CAD build for the part. Positions are in the model's coordinates, mm. A direction names the side the tool comes from. Give positions to 0.01 mm unless a question says otherwise; leave off trailing zeros. Loops run counter-clockwise (first coordinate to the right, second up) from the corner with the lowest first, then second, coordinate; pieces in that order, holes last. Notation, with made-up numbers: (13, 50.25) - (57, 50.25) arc R25 ccw to (57, 69.25) - close; hole circle Ø6 at (50.25, -31.75). An arc over 180 degrees is marked (long way). Return JSON: item names as keys, results as strings.
from build123d import *

# Parameters (mm, degrees)
SKETCH1_W           = 85
SKETCH1_H           = 76.5
SKETCH1_R           = 1.5
BOSS_EXTRUDE1_DEPTH = 10
SKETCH2_W           = 7
SKETCH2_H           = 7
BOSS_EXTRUDE2_DEPTH = 10


with BuildPart() as part:
    # Sketch1 → Boss-Extrude1 (new body)
    with BuildSketch(Plane(origin=(0, 0, 0), x_dir=(1, 0, 0), z_dir=(0, 1, 0))):
        Rectangle(SKETCH1_W, SKETCH1_H)
        with Locations(Location((-29.5, 25.25, 0), (0, 0, 270))):
            Circle(SKETCH1_R, mode=Mode.SUBTRACT)
        with Locations(Location((-29.5, -25.25, 0), (0, 0, 270))):
            Circle(SKETCH1_R, mode=Mode.SUBTRACT)
        with Locations(Location((29.5, -25.25, 0), (0, 0, 270))):
            Circle(SKETCH1_R, mode=Mode.SUBTRACT)
        with Locations(Location((29.5, 25.25, 0), (0, 0, 270))):
            Circle(SKETCH1_R, mode=Mode.SUBTRACT)
    extrude(amount=BOSS_EXTRUDE1_DEPTH)

    # Sketch2 → Boss-Extrude2 (add)
    with BuildSketch(Plane(origin=(0, 10, 0), x_dir=(1, 0, 0), z_dir=(0, 1, 0))):
        with Locations((-39, 34.75)):
            Rectangle(SKETCH2_W, SKETCH2_H)
        with Locations((39, 34.75)):
            Rectangle(SKETCH2_W, SKETCH2_H)
        with Locations((-39, -34.75)):
            Rectangle(SKETCH2_W, SKETCH2_H)
        with Locations((39, -34.75)):
            Rectangle(SKETCH2_W, SKETCH2_H)
    extrude(amount=BOSS_EXTRUDE2_DEPTH)


solid = part.part
1. Drop flat-ended pins along their axis: P1, Ø3, axis at y = 13, z = 18, coming from the -X side; P2, Ø3.5, axis at x = -29.5, z = 25.25, coming from the +Y side; P3, Ø10, axis at x = -8.5, z = 15, coming from the -Y side. Give the stop position or say it passes through.
Values follow:
{"P1": "passes through", "P2": "stops at y = 10", "P3": "stops at y = 0"}
2. Pull direction Z, two halves, no side cores. Call faces 1 (the face through (-1, 8, 38.25)), 2 (the face through (30.51, 4.93, -26.36)), 3 (the face through (-39, 15, -31.25)), 4 (the face through (-39, 20, -35)): +Z half, -Z half, draft (parallel to the pull), parting line (faces both ways), or undercut.
Values follow:
{"face 1": "+Z half", "face 2": "undercut", "face 3": "undercut", "face 4": "draft"}
3. Cut at C-C, the plane x = 29.5. Write the cut outline in (y, z), plus the area to 3 significant figures.
Values follow:
{"outline": "(0, -38.25) - (10, -38.25) - (10, -26.75) - (0, -26.75) - close; (0, -23.75) - (10, -23.75) - (10, 23.75) - (0, 23.75) - close; (0, 26.75) - (10, 26.75) - (10, 38.25) - (0, 38.25) - close", "area": "705 mm²"}
4. Drill centre lines: probe 1 along X at (y, z) = (6.75, -25.25); probe 2 along Y at (x, z) = (22, -23); probe 3 along X at (y, z) = (3.5, 24). Where is each one in solid material? Low to high.
Values follow:
{"probe 1": "x = -42.5 to -31, -28 to 28, 31 to 42.5", "probe 2": "y = 0 to 10", "probe 3": "x = -42.5 to -30.33, -28.67 to 28.67, 30.33 to 42.5"}
5. Cut at B-B, the plane z = -25.25. Write the cut outline in (x, y), plus the area to 3 significant figures.
Values follow:
{"outline": "(-42.5, 0) - (-31, 0) - (-31, 10) - (-42.5, 10) - close; (-28, 0) - (28, 0) - (28, 10) - (-28, 10) - close; (31, 0) - (42.5, 0) - (42.5, 10) - (31, 10) - close", "area": "790 mm²"}
6. Which spindle directions (+Z, -Z, +X, -X, +Y, -Y) get a long thin tool onto all of the face, cutting with end or side? Do faces 5 (the face through (35.5, 15, 35)), 6 (the face through (-39, 20, 35)), 7 (the face through (39, 15, 31.25)). Say none if no direction does.
Values follow:
{"face 5": "+Z, -Z, +Y", "face 6": "+Z, -Z, +X, -X, +Y", "face 7": "+X, -X, +Y"}
7. Cut at A-A, the plane y = 13. Write the cut outline in (x, z), plus the area to 3 significant figures.
Values follow:
{"outline": "(-42.5, -38.25) - (-35.5, -38.25) - (-35.5, -31.25) - (-42.5, -31.25) - close; (-42.5, 31.25) - (-35.5, 31.25) - (-35.5, 38.25) - (-42.5, 38.25) - close; (35.5, -38.25) - (42.5, -38.25) - (42.5, -31.25) - (35.5, -31.25) - close; (35.5, 31.25) - (42.5, 31.25) - (42.5, 38.25) - (35.5, 38.25) - close", "area": "196 mm²"}
8. Cut at D-D, the plane z = 33. Write the cut outline in (x, y).
Values follow:
{"outline": "(-42.5, 0) - (42.5, 0) - (42.5, 20) - (35.5, 20) - (35.5, 10) - (-35.5, 10) - (-35.5, 20) - (-42.5, 20) - close"}
